```python
from build123d import *

# Parameters (mm, degrees)
CUT_EXTRUDE1_DEPTH = 17.867127793
FILLET1_R          = 0.7
FILLET2_R          = 0.3


with BuildPart() as part:
    # Sketch2 → Revolve1 (revolve)
    with BuildSketch(Plane.XY, mode=Mode.PRIVATE) as revolve1_sk:
        Polygon((0, 0), (10.5, 0), (10.5, -1.5), (7.5, -1.5), (7.291240349, -2.985402103), (6.942652064, -2.936411215), (6.803478963, -3.926679283), (6.972213603, -3.950393391), (6.972213603, -4.374297025), (6.861946509, -4.75677404), (6.690208868, -4.732637888), (6.568289136, -5.600141858), (6.906531053, -5.722750977), (6.586484574, -8), (0, -8), align=None)
    revolve(revolve1_sk.sketch.rotate(Axis((0, 0, 0), (0, 1, 0)), 90), axis=Axis((0, 0, 0), (0, 1, 0)))

    # Sketch1 → Cut-Extrude1 (cut, through all)
    with BuildSketch(Plane(origin=(0, 0, 0), x_dir=(1, 0, 0), z_dir=(0, 1, 0))):
        with BuildLine():
            Line((-0.99, 0.99), (-2.284731932, 0.99))
            ThreePointArc((-2.284731932, 0.99), (-2.49, 0), (-2.284731932, -0.99))
            Line((-2.284731932, -0.99), (-0.99, -0.99))
            Line((-0.99, -0.99), (-0.99, -2.284731932))
            ThreePointArc((-0.99, -2.284731932), (0, -2.49), (0.99, -2.284731932))
            Line((0.99, -2.284731932), (0.99, -0.99))
            Line((0.99, -0.99), (2.284249826, -0.99))
            ThreePointArc((2.284249826, -0.99), (2.489557645, 0), (2.284249826, 0.99))
            Line((2.284249826, 0.99), (0.99, 0.99))
            Line((0.99, 0.99), (0.99, 2.28753254))
            ThreePointArc((0.99, 2.28753254), (0, 2.492569984), (-0.99, 2.28753254))
            Line((-0.99, 2.28753254), (-0.99, 0.99))
        make_face()
    extrude(amount=-CUT_EXTRUDE1_DEPTH, mode=Mode.SUBTRACT)

    # Fillet1
    fillet1_edges = [part.edges().sort_by_distance(p)[0] for p in [
        (-0.99, -4, -0.99),
        (0.99, -4, -0.99),
        (0.99, -4, 0.99),
        (-0.99, -4, 0.99),
    ]]
    fillet(fillet1_edges, radius=FILLET1_R)

    # Fillet2
    fillet2_edges = [part.edges().sort_by_distance(p)[0] for p in [
        (0, -1.5, 7.5),
        (0, -1.5, 10.5),
        (0, 0, 10.5),
    ]]
    fillet(fillet2_edges, radius=FILLET2_R)


solid = part.part
```
Geometry check sheet. Reference: the model listing, model coordinates, mm. A direction names the side the tool comes from. Coordinates: 2 decimals unless noted, no trailing zeros. Write each loop counter-clockwise with the first axis right and the second up, starting at its lowest first coordinate (ties: lowest second). Pieces come first, ordered by that corner, then holes. Notation, with made-up numbers: M -14,4 L 34,4 A30 cw 34,31 Z; hole C 82,66.25 d1. An arc over 180 degrees is marked long. One line per item, written item: value. Start each with the question number.
(1) Depth check by flat-ended pin: pin 1 (0.7 mm diameter, centred on x = -2, y = -5.5, fed in from +Z); pin 2 (0.5 mm diameter, centred on x = 2, y = -4.5, fed in from -Z); pin 3 (1.5 mm diameter, centred on x = 6, y = -1.5, fed in from +Z). Enter the tip coordinate at first touch or a pass-through.
(2) Tool access check on faces 1 (the face through (-8, -1.5, 2)), 2 (the face through (2, 0, 2)), 3 (the face through (2.49, -3.94, 0.01)). Record the directions out of +Z, -Z, +X, -X, +Y, -Y that give a thin tool (end or side, any length) a straight path to the whole face; none if there is none.
(3) Scan lines: line 1 along X through (y, z) = (-4.25, 1.75); line 2 along X through (y, z) = (-4.5, 0.25); line 3 along Y through (x, z) = (-5.25, -7.25). Record each from-to range of solid material in increasing order. Write a range as [from, to].
(4) Sectioned sample at A-A, the plane y = -0.75. Enter the section's corners in (x, z).
Filled sheet:
1. pin 1: z = 6.69
1. pin 2: z = -6.74
1. pin 3: z = 9.06
2. face 1: -Y
2. face 2: +Z, -Z, +X, -X, +Y
2. face 3: +Y, -Y
3. line 1: [-6.75, -0.99], [0.99, 6.75]
3. line 2: [-6.93, -2.48], [2.48, 6.93]
3. line 3: [-1.5, 0]
4. outline: C 0,0 d21; hole M -2.28,-0.99 L -1.69,-0.99 A0.7 cw -0.99,-1.69 L -0.99,-2.29 A2.49 ccw 0.99,-2.29 L 0.99,-1.69 A0.7 cw 1.69,-0.99 L 2.28,-0.99 A2.49 ccw 2.28,0.99 L 1.69,0.99 A0.7 cw 0.99,1.69 L 0.99,2.28 A2.49 ccw -0.99,2.28 L -0.99,1.69 A0.7 cw -1.69,0.99 L -2.28,0.99 A2.49 ccw Z
